Geometry: final body of the model. Coordinates: model frame, mm. Face numbers are marked on the shaded views. A direction names the side the tool comes from. Give positions to 0.01 mm unless a question says otherwise; leave off trailing zeros. Write each loop counter-clockwise with the first axis right and the second up, starting at its lowest first coordinate (ties: lowest second). Pieces come first, ordered by that corner, then holes. Notation, with made-up numbers: (-28, 22) -> (-8, 22) arc R31 ccw to (-8, 56) -> close; hole circle Ø6 at (19.25, 68.25). An arc over 180 degrees is marked (long way). Answer in a Markdown table with one row per item. Add a question column.
from build123d import *

# Parameters (mm, degrees)
SKETCH_1_W          = 110
SKETCH_1_H          = 100
EXTRUDE_1_DEPTH     = 25
SKETCH_2_W          = 110
SKETCH_2_H          = 25
EXTRUDE_2_DEPTH     = 25
SKETCH_3_W          = 40
SKETCH_3_H          = 35
CUT_EXTRUDE_1_DEPTH = 79.421935707
RIB_1_REACH         = 91.582
SKETCH_4_WALL_W     = 228.334634332
SKETCH_4_WALL_H     = 15
SKETCH_5_R          = 7
CUT_EXTRUDE_2_DEPTH = 90.582364336


with BuildPart() as part:
    # Эскиз1 → Бобышка-Вытянуть1 (new body)
    with BuildSketch(Plane(origin=(0, 0, 0), x_dir=(1, 0, 0), z_dir=(0, 1, 0))):
        Rectangle(SKETCH_1_W, SKETCH_1_H)
    extrude(amount=EXTRUDE_1_DEPTH)

    # Эскиз2 → Бобышка-Вытянуть2 (add)
    with BuildSketch(Plane(origin=(0, 25, 0), x_dir=(1, 0, 0), z_dir=(0, 1, 0))):
        with Locations((0, 37.5)):
            Rectangle(SKETCH_2_W, SKETCH_2_H)
    extrude(amount=EXTRUDE_2_DEPTH)

    # Эскиз3 → Вырез-Вытянуть1 (cut, through all)
    with BuildSketch(Plane(origin=(0, 25, 0), x_dir=(1, 0, 0), z_dir=(0, 1, 0))):
        with Locations((0, -32.5)):
            Rectangle(SKETCH_3_W, SKETCH_3_H)
    extrude(amount=-CUT_EXTRUDE_1_DEPTH, mode=Mode.SUBTRACT)

    # Эскиз4 wall → Ребро1 (add, up to next)
    with BuildSketch(Plane(origin=(0, 37.5, -5), x_dir=(0, -0.529998940003, 0.847998304005), z_dir=(0, -0.847998304005, -0.529998940003)), mode=Mode.PRIVATE) as rib_1_sk1:
        Rectangle(SKETCH_4_WALL_W, SKETCH_4_WALL_H)
    rib_1_tool1 = extrude(rib_1_sk1.sketch, amount=RIB_1_REACH, mode=Mode.PRIVATE) - part.part
    add(rib_1_tool1.solids().sort_by_distance((0, 37.5, -5))[0])

    # Эскиз5 → Вырез-Вытянуть2 (cut, through all)
    with BuildSketch(Plane(origin=(0, 50, 0), x_dir=(1, 0, 0), z_dir=(0, 1, 0))):
        with Locations(Location((0, 37.5, 0), (0, 0, 270))):
            Circle(SKETCH_5_R)
    extrude(amount=-CUT_EXTRUDE_2_DEPTH, mode=Mode.SUBTRACT)


solid = part.part
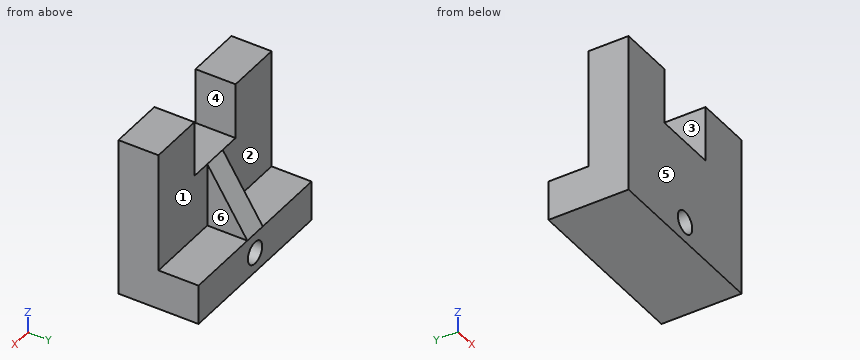
Q1. Section A-A on z = -37.5. Return loops of the section in (x, y).
Q2. Section C-C on x = 0. Return loops of the section in (y, z).
Q3. Line query: probe 1 along X at (y, z) = (34, -37); probe 2 along X at (y, z) = (5, 24.5); probe 3 along Z at (x, y) = (-43.5, 33). Output: solid intervals per line, ascending. Write a range as from..to.
Q4. Section D-D on z = 32.5. Return loops of the section in (x, y), and give its area (3 significant figures).
Q5. Pull-direction query (X, two-part tool) for the marked faces 4, 5 and 6; classes: +X half, -X half, draft (parallel to the pull), parting line (faces both ways), or undercut.
Q6. Access query for the marked faces 1, 2 and 3. Directions: +Z, -Z, +X, -X, +Y, -Y. A direction counts if a zero-diameter tool reaches every point of the face in a straight line with its end or side. Return the directions, or none.
Q7. Section B-B on y = 30.5. Return loops of the section in (x, z), and give its area (3 significant figures).
Q8. Contact query for flat-ended pins moving along their axis: pin 1 Ø12.5 at (x, y) = (-39.5, 41.5) entering from +Z; pin 2 Ø8.5 at (x, z) = (0, -37.5) entering from +Y; pin 3 Ø7.5 at (x, y) = (-10, 10.5) entering from +Z; pin 4 Ø14 at (x, z) = (-30, 30.5) entering from +Y. Output: stop coordinate, or through.
Checks:
| question | item | result |
|---|---|---|
| 1 | outline | (-55, 0) -> (-7, 0) -> (-7, 50) -> (-55, 50) -> close; (7, 0) -> (55, 0) -> (55, 50) -> (7, 50) -> close |
| 2 | outline | (0, -50) -> (50, -50) -> (50, -44.5) -> (0, -44.5) -> close; (0, -30.5) -> (50, -30.5) -> (50, -25) -> (25, 15) -> (0, 15) -> close |
| 3 | probe 1 | -55..-6.98, 6.98..55 |
| 3 | probe 2 | -55..-20, 20..55 |
| 3 | probe 3 | -50..-25 |
| 4 | outline | (-55, 0) -> (-20, 0) -> (-20, 25) -> (-55, 25) -> close; (20, 0) -> (55, 0) -> (55, 25) -> (20, 25) -> close |
| 4 | area | 1,750 mm^2 |
| 5 | face 4 | undercut |
| 5 | face 5 | draft |
| 5 | face 6 | +X half |
| 6 | face 1 | +Z, +X, +Y |
| 6 | face 2 | +Z, -X, +Y |
| 6 | face 3 | +Z, +Y, -Y |
| 7 | outline | (-55, -50) -> (55, -50) -> (55, -25) -> (7.5, -25) -> (7.5, 6.2) -> (-7.5, 6.2) -> (-7.5, -25) -> (-55, -25) -> close; hole circle Ø14 at (0, -37.5) |
| 7 | area | 3,060 mm^2 |
| 8 | pin 1 | z = -25 |
| 8 | pin 2 | through |
| 8 | pin 3 | z = 15 |
| 8 | pin 4 | y = 25 |
